Part model, mm, in its own coordinate system. Give positions to 0.01 mm unless a question says otherwise; leave off trailing zeros. Order: outer loops, then holes, each group sorted by start corner. A loop starts at its lowest first (then second) coordinate and runs counter-clockwise, first axis right, second up.
from build123d import *

# Parameters (mm, degrees)
SKETCH_R           = 7.5
SKETCH_R_2         = 3.6
PAD_DEPTH          = 45
SKETCH001_W        = 1
SKETCH001_H        = 2
POCKET_DEPTH       = 45
POLARPATTERN_COUNT = 16


with BuildPart() as part:
    # Sketch → Pad (new body)
    with BuildSketch(Plane.XY):
        Circle(SKETCH_R)
        Circle(SKETCH_R_2, mode=Mode.SUBTRACT)
    extrude(amount=PAD_DEPTH)

    # Sketch001 (on Face4 of Pad) → Pocket (cut)
    with BuildSketch(Plane.XY.offset(45)):
        with Locations((0, 4.565109)):
            Rectangle(SKETCH001_W, SKETCH001_H)
    pocket = extrude(amount=-POCKET_DEPTH, mode=Mode.SUBTRACT)

    # PolarPattern: Pocket ×16 about axis
    polarpattern_axis = Axis((0, 0, 45), (0, 0, 1))
    for i in range(1, POLARPATTERN_COUNT):
        add(pocket.rotate(polarpattern_axis, i * 360 / POLARPATTERN_COUNT), mode=Mode.SUBTRACT)


solid = part.part
Item 1: Pull direction X, two halves, no side cores. Call faces 1 (the face through (-7.493, 0.33, 22.185)), 2 (the face through (-0.5, 5, 23)): released by +X, released by -X, zero draft, split by the parting line, or undercut.
Item 2: Band-saw the part on A-A on x = 0. List the corners of the cut face in (y, z), plus the area to 3 significant figures.
Item 3: Drill centre lines: probe 1 along Y at (x, z) = (-4.75, 43); probe 2 along X at (y, z) = (-3, 4.5); probe 3 along X at (y, z) = (2.25, 23). Where is each one in solid material? Low to high.
Item 4: Drop flat-ended pins along their axis: P1, Ø5, axis at x = -1, y = 1.5, coming from the -Z side; P2, Ø2, axis at y = 4.5, z = 27.5, coming from the +X side; P3, Ø5, axis at y = -4, z = 17, coming from the +X side; P4, Ø0.6, axis at x = 4.5, z = 17, coming from the +Y side. Give the stop position or say it passes through.
Working result:
1. face 1: split by the parting line
1. face 2: undercut
2. outline: (-7.5, 0) - (-5.57, 0) - (-5.57, 45) - (-7.5, 45) - close; (5.57, 0) - (7.5, 0) - (7.5, 45) - (5.57, 45) - close
2. area: 174 mm2
3. probe 1: y = -5.8 to -2.51, -1.43 to -0.5, 0.5 to 1.43, 2.51 to 5.8
3. probe 2: x = -6.87 to -3.71, -2.29 to -1.99, 1.99 to 2.29, 3.71 to 6.87
3. probe 3: x = -7.15 to -5.09, -4.13 to -2.96, 2.96 to 4.13, 5.09 to 7.15
4. P1: stops at z = 0
4. P2: stops at x = 6.63
4. P3: stops at x = 7.35
4. P4: stops at y = 6.21
